Autodesk Inventor part; units mm, degrees
ref_plane "YZ Plane" through (0, 0, 0) normal (1, 0, 0) x (0, 1, 0)
ref_plane "XZ Plane" through (0, 0, 0) normal (0, 1, 0) x (-1, 0, 0)
ref_plane "XY Plane" through (0, 0, 0) normal (0, 0, 1) x (1, 0, 0)
sketch "Sketch1" plane through (0, 0, 0) normal (0, 0, 1) x (1, 0, 0)
  line L0 (-6.35, -3.6662) -> (-6.35, 3.6662)
  line L1 (-6.35, 3.6662) -> (0, 7.3323)
  line L2 (0, 7.3323) -> (6.35, 3.6662)
  line L3 (6.35, 3.6662) -> (6.35, -3.6662)
  line L4 (6.35, -3.6662) -> (0, -7.3323)
  line L5 (0, -7.3323) -> (-6.35, -3.6662)
  point P0 (0, 0)
  point P1 (0, 0)
  dimension "Size" = 12.7
extrude "Extrusion1" add sketch "Sketch1" along normal mid plane 66.675
sketch "Sketch3" plane through (0, 0, 33.3375) normal (0, 0, 1) x (1, 0, 0)
  line L0 (-6.35, 3.6662) -> (0, 7.3323) construction
  line L1 (0, 7.3323) -> (6.35, 3.6662) construction
  line L2 (6.35, 3.6662) -> (6.35, -3.6662) construction
  line L3 (6.35, -3.6662) -> (0, -7.3323) construction
  line L4 (0, -7.3323) -> (-6.35, -3.6662) construction
  line L5 (-6.35, -3.6662) -> (-6.35, 3.6662) construction
  point P0 (0, 0)
hole "Hole1" at (0, 0, 33.3375) direction (0, 0, -1) diameter 5.1054 end through all
sketch "Sketch4" plane through (0, 0, 33.3375) normal (0, 0, 1) x (1, 0, 0)
  circle A0 centre (0, 0) radius 2.5527 construction
  line L0 (-6.35, 3.6662) -> (0, 7.3323) construction
  line L1 (0, 7.3323) -> (6.35, 3.6662) construction
  line L2 (6.35, 3.6662) -> (6.35, -3.6662) construction
  line L3 (6.35, -3.6662) -> (0, -7.3323) construction
  line L4 (0, -7.3323) -> (-6.35, -3.6662) construction
  line L5 (-6.35, -3.6662) -> (-6.35, 3.6662) construction
  circle A1 centre (0, 0) radius 6.8771
  circle A2 centre (0, 0) radius 8.89
  dimension "thunder" = 13.7541
  dimension "d16" = 17.78
extrude "Extrusion3" cut sketch "Sketch4" against normal through all
sketch "Sketch5" plane through (0, 0, 33.3375) normal (0, 0, 1) x (1, 0, 0)
  circle A0 centre (0, 0) radius 2.5527
  circle A1 centre (0, 0) radius 6.35
  arc A2 (5.4616, -4.1791) -> (6.35, -2.6403) centre (0, 0) ccw
  line L0 (6.35, -2.6403) -> (6.35, 2.6403)
  arc A3 (6.35, 2.6403) -> (5.4616, 4.1791) centre (0, 0) ccw
  line L1 (5.4616, 4.1791) -> (0.8884, 6.8194)
  arc A4 (0.8884, 6.8194) -> (-0.8884, 6.8194) centre (0, 0) ccw
  line L2 (-0.8884, 6.8194) -> (-5.4616, 4.1791)
  arc A5 (-5.4616, 4.1791) -> (-6.35, 2.6403) centre (0, 0) ccw
  line L3 (-6.35, 2.6403) -> (-6.35, -2.6403)
  arc A6 (-6.35, -2.6403) -> (-5.4616, -4.1791) centre (0, 0) ccw
  line L4 (-5.4616, -4.1791) -> (-0.8884, -6.8194)
  arc A7 (-0.8884, -6.8194) -> (0.8884, -6.8194) centre (0, 0) ccw
  line L5 (0.8884, -6.8194) -> (5.4616, -4.1791)
  circle A8 centre (0, 0) radius 2.5527
  point P0 (3.175, -5.4993)
  point P1 (-3.175, -5.4993)
  point P2 (-6.35, 0)
  point P3 (-3.175, 5.4993)
  point P4 (3.175, 5.4993)
  point P5 (6.35, 0)
  dimension "d21" = 12.7
extrude "Extrusion4" cut sketch "Sketch5" against normal blind 7.9248 contours A0 | L0 A2 L5 A1 | A1 L1 A3 L0 | A1 L2 A4 L1 | L5 A7 L4 A1 | A1 L3 A5 L2 | L4 A6 L3 A1
mirror "Mirror2" about plane through (0, 0, 0) normal (0, 0, 1) of "Extrusion4"
equation "\"bearing\" = 25.4"
properties part number "GP10-011" material "Aluminum 6061"
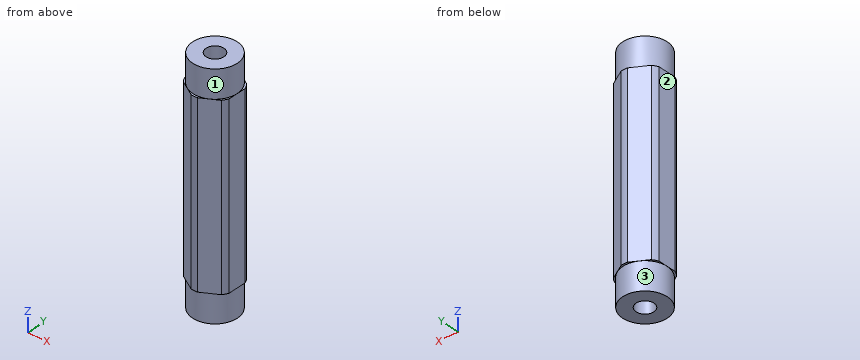
Design review of the part built by this model. Coordinates are the model's own, in mm. Face numbers are marked on the shaded views. A direction names the side the tool comes from. Coordinates: 2 decimals unless noted, no trailing zeros. Order: outer loops, then holes, each group sorted by start corner. A loop starts at its lowest first (then second) coordinate and runs counter-clockwise, first axis right, second up.
Item 1: For pin 1 Ø6 at (x, z) = (3.5, -12.5) entering from +Y, flat-tipped, find the tip position at first contact; note if it passes through.
Item 2: For line 1 (X direction, y = 0, z = 11); line 2 (Y direction, x = -1, z = -18); line 3 (X direction, y = -2.25, z = -30), list the stretches that pass through material, from the lowest coordinate up.
Item 3: Take a section at C-C, the plane z = -24. Write out the cut boundary in (x, y), then the cut area to 3 significant figures.
Item 4: Take a section at A-A, the plane y = 1.25. Write out the cut boundary in (x, z).
Item 5: Take a section at B-B, the plane x = 0. Write out the cut boundary in (y, z), then the cut area to 3 significant figures.
Item 6: For the marked faces 1, 2 and 3, list the 3-axis set-ups (+Z, -Z, +X, -X, +Y, -Y) from which the entire face can be reached by the end or side of a thin tool; tool diameter is ignored.
The answers:
1. pin 1: stops at y = 6.86
2. line 1: x = -6.35 to -2.55, 2.55 to 6.35
2. line 2: y = -6.75 to -2.35, 2.35 to 6.75
2. line 3: x = -5.94 to -1.21, 1.21 to 5.94
3. outline: (-6.35, -2.64) arc R6.88 ccw to (-5.46, -4.18) - (-0.89, -6.82) arc R6.88 ccw to (0.89, -6.82) - (5.46, -4.18) arc R6.88 ccw to (6.35, -2.64) - (6.35, 2.64) arc R6.88 ccw to (5.46, 4.18) - (0.89, 6.82) arc R6.88 ccw to (-0.89, 6.82) - (-5.46, 4.18) arc R6.88 ccw to (-6.35, 2.64) - close; hole circle Ø5.11 at (0, 0)
3. area: 117 mm2
4. outline: (-6.35, -25.41) - (-6.23, -25.41) - (-6.23, -33.34) - (-2.23, -33.34) - (-2.23, 33.34) - (-6.23, 33.34) - (-6.23, 25.41) - (-6.35, 25.41) - close; (2.23, -33.34) - (6.23, -33.34) - (6.23, -25.41) - (6.35, -25.41) - (6.35, 25.41) - (6.23, 25.41) - (6.23, 33.34) - (2.23, 33.34) - close
5. outline: (-6.88, -25.41) - (-6.35, -25.41) - (-6.35, -33.34) - (-2.55, -33.34) - (-2.55, 33.34) - (-6.35, 33.34) - (-6.35, 25.41) - (-6.88, 25.41) - close; (2.55, -33.34) - (6.35, -33.34) - (6.35, -25.41) - (6.88, -25.41) - (6.88, 25.41) - (6.35, 25.41) - (6.35, 33.34) - (2.55, 33.34) - close
5. area: 560 mm2
6. face 1: +Z
6. face 2: +Z, -Z, -X, +Y, -Y
6. face 3: -Z
